from build123d import *

# Parameters (mm, degrees)
CROQUIS1_W              = 62
CROQUIS1_H              = 62
SALIENTE_EXTRUIR1_DEPTH = 20
CORTAR_EXTRUIR1_DEPTH   = 17
CORTAR_EXTRUIR2_DEPTH   = 2
CORTAR_EXTRUIR3_START   = -18
CROQUIS4_R              = 1.5
CORTAR_EXTRUIR3_DEPTH   = 18
CROQUIS5_W              = 16
CROQUIS5_H              = 13
SALIENTE_EXTRUIR2_DEPTH = 8
CROQUIS6_W              = 11.961680629
CROQUIS6_H              = 9
CORTAR_EXTRUIR4_DEPTH   = 8
CROQUIS7_W              = 7
CROQUIS7_H              = 7
CORTAR_EXTRUIR5_DEPTH   = 1
CORTAR_EXTRUIR6_START   = -16
CROQUIS8_W              = 11.5
CROQUIS8_H              = 2.4
CORTAR_EXTRUIR6_DEPTH   = 16


with BuildPart() as part:
    # Croquis1 → Saliente-Extruir1 (new body)
    with BuildSketch(Plane.XY):
        with Locations((-78.537903487, 2.596858639)):
            Rectangle(CROQUIS1_W, CROQUIS1_H)
    extrude(amount=SALIENTE_EXTRUIR1_DEPTH)

    # Croquis2 → Cortar-Extruir1 (cut)
    with BuildSketch(Plane.XY.offset(20)):
        Polygon((-106.537903487, 27.596858639), (-106.537903487, -22.403141361), (-102.537903487, -22.403141361), (-102.537903487, -24.403141361), (-99.537903487, -24.403141361), (-99.537903487, -25.903141361), (-99.537903487, -27.403141361), (-54.537903487, -27.403141361), (-54.537903487, -25.903141361), (-54.537903487, -5.903141361), (-49.537903487, -5.903141361), (-49.537903487, 11.096858639), (-55.537903487, 11.096858639), (-55.537903487, 30.596858639), (-55.537903487, 31.596858639), (-69.537903487, 31.596858639), (-69.537903487, 29.596858639), (-72.537903487, 29.596858639), (-72.537903487, 27.596858639), (-75.537903487, 27.596858639), (-75.537903487, -22.403141361), (-76.537903487, -22.403141361), (-76.537903487, 27.596858639), (-80.537903487, 27.596858639), (-80.537903487, 29.596858639), (-102.537903487, 29.596858639), (-102.537903487, 27.596858639), align=None)
        Polygon((-92.037903487, 27.596858639), (-91.037903487, 27.596858639), (-91.037903487, -22.403141361), (-87.037903487, -22.403141361), (-87.037903487, -24.403141361), (-65.037903487, -24.403141361), (-65.037903487, -22.403141361), (-61.037903487, -22.403141361), (-61.037903487, 27.596858639), (-65.037903487, 27.596858639), (-65.037903487, 28.596858639), (-57.037903487, 28.596858639), (-57.037903487, -24.403141361), (-57.037903487, -25.403141361), (-96.037903487, -25.403141361), (-96.037903487, -24.403141361), (-96.037903487, -22.403141361), (-92.037903487, -22.403141361), align=None, mode=Mode.SUBTRACT)
    extrude(amount=-CORTAR_EXTRUIR1_DEPTH, mode=Mode.SUBTRACT)

    # Croquis3 → Cortar-Extruir2 (cut)
    with BuildSketch(Plane.XY.offset(20)):
        Polygon((-108.537903487, 27.596858639), (-108.537903487, 32.596858639), (-48.537903487, 32.596858639), (-48.537903487, -27.403141361), (-108.537903487, -27.403141361), align=None)
    extrude(amount=-CORTAR_EXTRUIR2_DEPTH, mode=Mode.SUBTRACT)

    # Croquis4 → Cortar-Extruir3 (cut)
    with BuildSketch(Plane.XY.offset(18).offset(CORTAR_EXTRUIR3_START)):
        with Locations((-106.037903487, 30.096858639)):
            Circle(CROQUIS4_R)
        with Locations((-51.037903487, 30.096858639)):
            Circle(CROQUIS4_R)
        with Locations((-51.037903487, -24.903141361)):
            Circle(CROQUIS4_R)
        with Locations((-106.037903487, -24.903141361)):
            Circle(CROQUIS4_R)
    extrude(amount=CORTAR_EXTRUIR3_DEPTH, mode=Mode.SUBTRACT)

    # Croquis5 → Saliente-Extruir2 (add)
    with BuildSketch(Plane.XZ.offset(28.403141361)):
        with Locations((-78.537903487, 10)):
            Rectangle(CROQUIS5_W, CROQUIS5_H)
    extrude(amount=SALIENTE_EXTRUIR2_DEPTH)

    # Croquis6 → Cortar-Extruir4 (cut)
    with BuildSketch(Plane.XZ.offset(36.403141361)):
        with Locations((-78.557063173, 10)):
            Rectangle(CROQUIS6_W, CROQUIS6_H)
    extrude(amount=-CORTAR_EXTRUIR4_DEPTH, mode=Mode.SUBTRACT)

    # Croquis7 → Cortar-Extruir5 (cut)
    with BuildSketch(Plane.XZ.offset(28.403141361)):
        with Locations((-80.037903487, 10)):
            Rectangle(CROQUIS7_W, CROQUIS7_H)
    extrude(amount=-CORTAR_EXTRUIR5_DEPTH, mode=Mode.SUBTRACT)

    # Croquis8 → Cortar-Extruir6 (cut)
    with BuildSketch(Plane(origin=(-70.537903487, 0, 0), x_dir=(0, 0, -1), z_dir=(1, 0, 0)).offset(CORTAR_EXTRUIR6_START)):
        with Locations((-10, -33.203141361)):
            Rectangle(CROQUIS8_W, CROQUIS8_H)
    extrude(amount=CORTAR_EXTRUIR6_DEPTH, mode=Mode.SUBTRACT)


solid = part.part
Can you work these out from the model? Positions are in its coordinate system, mm. A direction names the side the tool comes from. Round coordinates to 2 decimals unless told otherwise and drop trailing zeros. Write each loop counter-clockwise with the first axis right and the second up, starting at its lowest first coordinate (ties: lowest second). Pieces come first, ordered by that corner, then holes. Notation, with made-up numbers: M 47,14 L 88,14 A26 ccw 88,50 Z; hole C 25,3.25 d3. An arc over 180 degrees is marked long. Use a Markdown table: item, result.
Item 1: Which directions (+Z, -Z, +X, -X, +Y, -Y) give clear straight access to the entire face, cutting with the end or side of a thin tool? Please do faces 3 (the face through (-107.228, -25.816, 8.874)), 4 (the face through (-79, -30, 14.5)), 5 (the face through (-70.538, -31, 10)), 6 (the face through (-54.538, -17, 11)).
Found:
| item | result |
|---|---|
| face 3 | +Z, -Z |
| face 4 | -Y |
| face 5 | +Z, -Z, +X, -Y |
| face 6 | +Z |
Item 2: I want a section at C-C (z = 1.5). List the corners of the cut face in (x, y) for me, and give its area (3 significant figures).
Found:
| item | result |
|---|---|
| outline | M -109.54,-28.4 L -47.54,-28.4 L -47.54,33.6 L -109.54,33.6 Z; hole C -106.04,-24.9 d3; hole C -106.04,30.1 d3; hole C -51.04,-24.9 d3; hole C -51.04,30.1 d3 |
| area | 3,820 mm2 |
Item 3: If I drill on line 1 along X through (y, z) = (15, 4.25); line 2 along X through (y, z) = (-17, 4); line 3 along Y through (x, z) = (-89, 17.25), over which ranges is the centre line in solid material (lowest first)? Write a range as [from, to].
Found:
| item | result |
|---|---|
| line 1 | x = [-109.54, -106.54], [-92.04, -91.04], [-76.54, -75.54], [-61.04, -57.04], [-55.54, -47.54] |
| line 2 | x = [-109.54, -106.54], [-92.04, -91.04], [-76.54, -75.54], [-61.04, -57.04], [-54.54, -47.54] |
| line 3 | y = [-28.4, -27.4], [-25.4, -22.4], [29.6, 33.6] |
Item 4: We'd pull the mould along Z, two halves only. Please class faces 1 (the face through (-79, -33, 4.25)), 2 (the face through (-62, 31.597, 11)): released by +Z, released by -Z, zero draft, split by the parting line, or undercut.
Found:
| item | result |
|---|---|
| face 1 | undercut |
| face 2 | zero draft |
Item 5: I want a section at D-D (z = 7.75). State how many separate pieces and enclosed holes the cut face has, and give its area (3 significant figures).
Found:
| item | result |
|---|---|
| separate pieces | 4 |
| enclosed holes | 4 |
| area | 1,210 mm2 |
Item 6: I want a section at A-A (y = -2.5). List the corners of the cut face in (x, z) for me.
Found:
| item | result |
|---|---|
| outline | M -109.54,0 L -47.54,0 L -47.54,20 L -48.54,20 L -48.54,18 L -49.54,18 L -49.54,3 L -57.04,3 L -57.04,18 L -61.04,18 L -61.04,3 L -75.54,3 L -75.54,18 L -76.54,18 L -76.54,3 L -91.04,3 L -91.04,18 L -92.04,18 L -92.04,3 L -106.54,3 L -106.54,18 L -108.54,18 L -108.54,20 L -109.54,20 Z |
Item 7: For pin 1 Ø1 at (x, y) = (-81, 22) entering from +Z; pin 2 Ø8 at (x, z) = (-99, 14.5) entering from -Y; pin 3 Ø0.6 at (y, z) = (-35.5, 10.5) entering from -X, each with a flat end and sliding along its axis, tell me the tip position at first contact or that it passes through.
Found:
| item | result |
|---|---|
| pin 1 | stops at z = 3 |
| pin 2 | stops at y = -28.4 |
| pin 3 | stops at x = -86.54 |
